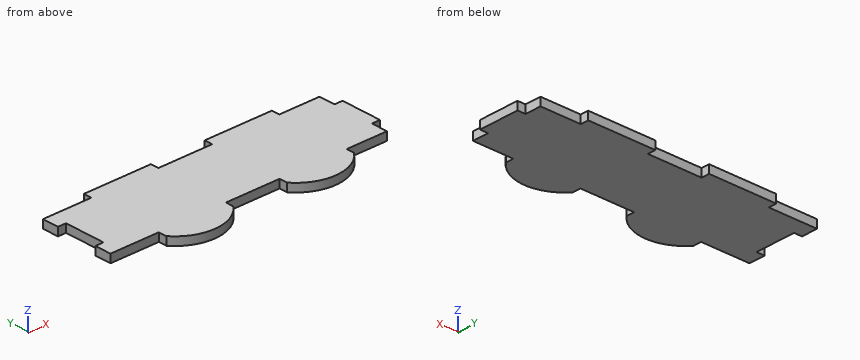
```python
from build123d import *

# Parameters (mm, degrees)
EXTRUDE_DEPTH = 3


with BuildPart() as part:
    # Sketch → Extrude (new body)
    with BuildSketch(Plane.XY):
        with BuildLine():
            Line((40, -6.37), (40, -9.37))
            ThreePointArc((15, -9.37), (27.5, -15.37), (40, -9.37))
            Line((15, -9.37), (15, -6.37))
            Line((15, -6.37), (0, -6.37))
            Line((-3, -6.37), (0, -6.37))
            Line((-3, -0.34), (-3, -6.37))
            Line((-3, -0.34), (0, -0.34))
            Line((0, 14.66), (0, -0.34))
            Line((0, 14.66), (-3, 14.66))
            Line((-3, 14.66), (-3, 20.66))
            Line((-3, 20.66), (0, 20.66))
            Line((0, 20.66), (15, 20.66))
            Line((15, 23.66), (15, 20.66))
            Line((40, 23.66), (15, 23.66))
            Line((40, 20.66), (40, 23.66))
            Line((40, 20.66), (60, 20.66))
            Line((60, 23.66), (60, 20.66))
            Line((85, 23.66), (60, 23.66))
            Line((85, 20.66), (85, 23.66))
            Line((85, 20.66), (100, 20.66))
            Line((100, 20.66), (100, 14.66))
            Line((100, 14.66), (103, 14.66))
            Line((103, 14.66), (103, -0.34))
            Line((103, -0.34), (100, -0.34))
            Line((100, -0.34), (100, -6.37))
            Line((100, -6.37), (85, -6.37))
            Line((85, -6.37), (85, -9.37))
            ThreePointArc((60, -9.37), (72.5, -15.37), (85, -9.37))
            Line((60, -9.37), (60, -6.37))
            Line((60, -6.37), (40, -6.37))
        make_face()
    extrude(amount=EXTRUDE_DEPTH)


solid = part.part
```
Part model, mm, in its own coordinate system. Give positions to 0.01 mm unless a question says otherwise; leave off trailing zeros. Write each loop counter-clockwise with the first axis right and the second up, starting at its lowest first coordinate (ties: lowest second). Pieces come first, ordered by that corner, then holes. Notation, with made-up numbers: M 72.5,77.5 L 98.5,77.5 A28 cw 98.5,104.5 Z; hole C 8.5,-35.75 d2. An arc over 180 degrees is marked long. Use CSV: the item, a comma, the result in double quotes.
Item 1: Slice it at B-B on z = 0.9. Write the cut outline in (x, y), plus the area to 3 significant figures.
Taken from the geometry:
outline,"M -3,-6.37 L 15,-6.37 L 15,-9.37 A16.02 ccw 40,-9.37 L 40,-6.37 L 60,-6.37 L 60,-9.37 A16.02 ccw 85,-9.37 L 85,-6.37 L 100,-6.37 L 100,-0.34 L 103,-0.34 L 103,14.66 L 100,14.66 L 100,20.66 L 85,20.66 L 85,23.66 L 60,23.66 L 60,20.66 L 40,20.66 L 40,23.66 L 15,23.66 L 15,20.66 L -3,20.66 L -3,14.66 L 0,14.66 L 0,-0.34 L -3,-0.34 Z"
area,"3,290 mm²"
Item 2: Drill centre lines: probe 1 along Y at (x, z) = (28, 1.55); probe 2 along X at (y, z) = (19, 2.2); probe 3 along X at (y, z) = (21.5, 1.8). Where is each one in solid material? Low to high.
Taken from the geometry:
probe 1,"y = -15.36 to 23.66"
probe 2,"x = -3 to 100"
probe 3,"x = 15 to 40, 60 to 85"
Item 3: Pin check, flat tips, straight feed: P1, Ø1.5, axis at x = 8.5, z = 2, coming from the +Y side; P2, Ø0.9, axis at y = 22.5, z = 1, coming from the +X side; P3, Ø1.5, axis at y = 17.5, z = 1, coming from the +X side. Stop position of each tip, or through.
Taken from the geometry:
P1,"stops at y = 20.66"
P2,"stops at x = 85"
P3,"stops at x = 100"
Item 4: Slice it at C-C on y = 7.5. Write the cut outline in (x, z).
Taken from the geometry:
outline,"M 0,0 L 103,0 L 103,3 L 0,3 Z"
Item 5: Slice it at A-A on y = -12. Write the cut outline in (x, z), plus the area to 3 significant figures.
Taken from the geometry:
outline,"M 17.67,0 L 37.33,0 L 37.33,3 L 17.67,3 Z; M 62.67,0 L 82.33,0 L 82.33,3 L 62.67,3 Z"
area,"118 mm²"
Item 6: Slice it at D-D on x = 89.5. Write the cut outline in (y, z).
Taken from the geometry:
outline,"M -6.37,0 L 20.66,0 L 20.66,3 L -6.37,3 Z"
